Geometry: see drawing. Coordinates: mm, zero at the bounding-box minimum. Give positions to 0.01 mm unless a question says otherwise; leave off trailing zeros. Loops run counter-clockwise (first coordinate to the right, second up) from the corner with the lowest first, then second, coordinate; pieces in that order, holes last. Notation, with made-up numbers: M -3,-34.75 L 23,-34.75 A22 ccw 23,1.25 Z; hole C -18.5,60.5 d7. An arc over 180 degrees is marked long. Put each result on its own line as item: value.
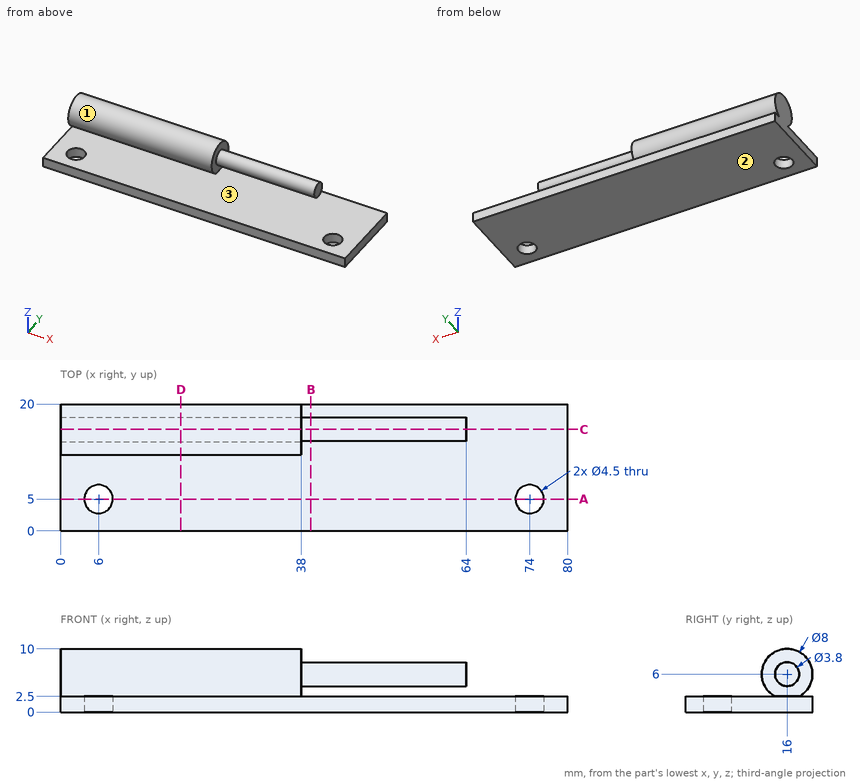
Item 1: Mould query, pull axis Z, two halves, no side actions, for the marked faces 1, 2 and 3. Classes: pulls with the +Z half, pulls with the -Z half, needs draft (parallel to the pull), parting line crosses it, or undercut.
Output values:
face 1: undercut
face 2: pulls with the -Z half
face 3: undercut
Item 2: Line query: probe 1 along X at (y, z) = (5, 0.65); probe 2 along Y at (x, z) = (6, 0.5); probe 3 along Z at (x, y) = (41.5, 5.25). Output: solid intervals per line, ascending. Write a range as [from, to].
Output values:
probe 1: [0, 3.75], [8.25, 71.75], [76.25, 80]
probe 2: [0, 2.75], [7.25, 20]
probe 3: [0, 2.5]
Item 3: Section C-C on y = 16. Output: boundary loops of the cut face in (x, z), then the cut area to 3 significant figures.
Output values:
outline: M 0,0 L 80,0 L 80,2.5 L 38,2.5 L 38,4.1 L 64,4.1 L 64,7.9 L 38,7.9 L 38,10 L 0,10 Z
area: 584 mm²
Item 4: Section D-D on x = 19. Output: boundary loops of the cut face in (y, z).
Output values:
outline: M 0,0 L 20,0 L 20,2.5 L 17.94,2.5 A4 ccw long 14.06,2.5 L 0,2.5 Z
Item 5: Section B-B on x = 39.5. Output: boundary loops of the cut face in (y, z), then the cut area to 3 significant figures.
Output values:
outline: M 0,0 L 20,0 L 20,2.5 L 0,2.5 Z; C 16,6 d3.8
area: 61.3 mm²
Item 6: Section A-A on y = 5. Output: boundary loops of the cut face in (x, z).
Output values:
outline: M 0,0 L 3.75,0 L 3.75,2.5 L 0,2.5 Z; M 8.25,0 L 71.75,0 L 71.75,2.5 L 8.25,2.5 Z; M 76.25,0 L 80,0 L 80,2.5 L 76.25,2.5 Z
Item 7: Pin query (flat end, axial travel): pin 1 Ø1.5 at (x, z) = (40.5, 4) entering from -Y; pin 2 Ø3 at (y, z) = (16.5, 5.5) entering from +X; pin 3 Ø7 at (x, y) = (6, 5) entering from +Z; pin 4 Ø2.5 at (x, y) = (74, 5) entering from -Z. Return the tip coordinate at first contact, or that it passes through.
Output values:
pin 1: y = 14.57
pin 2: x = 64
pin 3: z = 2.5
pin 4: through
